from build123d import *

# Parameters (mm, degrees)
SKETCH_1_W          = 550
SKETCH_1_H          = 18
SKETCH_1_R          = 2.75
EXTRUDE_1_DEPTH     = 10
FILLET_1_R          = 5
SKETCH_2_R          = 2.75
CUT_EXTRUDE_1_DEPTH = 10


with BuildPart() as part:
    # 草图1 → 凸台-拉伸1 (new body)
    with BuildSketch(Plane.XY):
        with Locations((275, -9)):
            Rectangle(SKETCH_1_W, SKETCH_1_H)
        with Locations((15, -9)):
            Circle(SKETCH_1_R, mode=Mode.SUBTRACT)
        with Locations((85, -9)):
            Circle(SKETCH_1_R, mode=Mode.SUBTRACT)
        with Locations(Location((465, -9, 0), (0, 0, 180))):
            Circle(SKETCH_1_R, mode=Mode.SUBTRACT)
        with Locations(Location((535, -9, 0), (0, 0, 180))):
            Circle(SKETCH_1_R, mode=Mode.SUBTRACT)
    extrude(amount=EXTRUDE_1_DEPTH)

    # 圆角1
    fillet_1_edges = [part.edges().sort_by_distance(p)[0] for p in [
        (0, 0, 5),
        (550, 0, 5),
        (550, -18, 5),
        (0, -18, 5),
    ]]
    fillet(fillet_1_edges, radius=FILLET_1_R)

    # 草图2 → 切除-拉伸1 (cut)
    with BuildSketch(Plane.XY.offset(10)):
        with Locations((385, -9)):
            Circle(SKETCH_2_R)
        with Locations(Location((165, -9, 0), (0, 0, 180))):
            Circle(SKETCH_2_R)
    extrude(amount=-CUT_EXTRUDE_1_DEPTH, mode=Mode.SUBTRACT)


solid = part.part
Could you check a few things on this model? Use its own coordinates, in mm. Give positions to 0.01 mm unless a question says otherwise; leave off trailing zeros. Order: outer loops, then holes, each group sorted by start corner. A loop starts at its lowest first (then second) coordinate and runs counter-clockwise, first axis right, second up.
Item 1: I need wall thicknesses on line 1 (Y direction, x = 385, z = 7.5); line 2 (X direction, y = -4.5, z = 7.5); line 3 (X direction, y = -14, z = 3). Which ranges of each line are inside material? Lowest first, please.
Item 2: I'm going to push a flat-ended pin straight in: pin 1 (3.5 mm diameter, centred on x = 165, y = -9, fed in from -Z). Where does the tip first touch, or does it pass through?
Item 3: If we section it at B-B, the plane z = 5: Write out the boundary of the cut face in (x, y).
Item 4: If we section it at A-A, the plane y = -9: Write out the boundary of the cut face in (x, z), plus the area to 3 significant figures.
Values:
1. line 1: y = -18 to -11.75, -6.25 to 0
1. line 2: x = 0.03 to 549.97
1. line 3: x = 0.1 to 549.9
2. pin 1: passes through
3. outline: (0, -13) arc R5 ccw to (5, -18) - (545, -18) arc R5 ccw to (550, -13) - (550, -5) arc R5 ccw to (545, 0) - (5, 0) arc R5 ccw to (0, -5) - close; hole circle Ø5.5 at (15, -9); hole circle Ø5.5 at (85, -9); hole circle Ø5.5 at (165, -9); hole circle Ø5.5 at (385, -9); hole circle Ø5.5 at (465, -9); hole circle Ø5.5 at (535, -9)
4. outline: (0, 0) - (12.25, 0) - (12.25, 10) - (0, 10) - close; (17.75, 0) - (82.25, 0) - (82.25, 10) - (17.75, 10) - close; (87.75, 0) - (162.25, 0) - (162.25, 10) - (87.75, 10) - close; (167.75, 0) - (382.25, 0) - (382.25, 10) - (167.75, 10) - close; (387.75, 0) - (462.25, 0) - (462.25, 10) - (387.75, 10) - close; (467.75, 0) - (532.25, 0) - (532.25, 10) - (467.75, 10) - close; (537.75, 0) - (550, 0) - (550, 10) - (537.75, 10) - close
4. area: 5,170 mm2
